```python
from build123d import *

# Parameters (mm, degrees)
SKETCH1_W           = 140
SKETCH1_H           = 70
BOSS_EXTRUDE1_DEPTH = 140
SKETCH2_W           = 134
SKETCH2_H           = 64
CUT_EXTRUDE1_DEPTH  = 133
SKETCH5_W           = 75.000260503
SKETCH5_H           = 36.846473491
BOSS_EXTRUDE3_DEPTH = 20
SKETCH6_W           = 5.75
SKETCH6_H           = 13
CUT_EXTRUDE2_DEPTH  = 3
SKETCH9_W           = 17
SKETCH9_H           = 30.85
CUT_EXTRUDE3_DEPTH  = 67
SKETCH11_W          = 140
SKETCH11_H          = 140
BOSS_EXTRUDE5_DEPTH = 5
SKETCH15_W          = 134
SKETCH15_H          = 4.072298399
CUT_EXTRUDE4_DEPTH  = 137


with BuildPart() as part:
    # Sketch1 → Boss-Extrude1 (new body)
    with BuildSketch(Plane(origin=(0, 0, 0), x_dir=(1, 0, 0), z_dir=(0, 1, 0))):
        with Locations((-46.886792453, 23.003144654)):
            Rectangle(SKETCH1_W, SKETCH1_H)
    extrude(amount=BOSS_EXTRUDE1_DEPTH)

    # Sketch2 → Cut-Extrude1 (cut)
    with BuildSketch(Plane(origin=(0, 140, 0), x_dir=(1, 0, 0), z_dir=(0, 1, 0))):
        with Locations((-46.932929257, 23.070074841)):
            Rectangle(SKETCH2_W, SKETCH2_H)
    extrude(amount=-CUT_EXTRUDE1_DEPTH, mode=Mode.SUBTRACT)

    # Sketch5 → Boss-Extrude3 (add)
    with BuildSketch(Plane.ZY.offset(116.886792453)):
        with Locations((-20.503014402, 18.423236746)):
            Rectangle(SKETCH5_W, SKETCH5_H)
    extrude(amount=BOSS_EXTRUDE3_DEPTH)

    # Sketch6 → Cut-Extrude2 (cut)
    with BuildSketch(Plane(origin=(0, 0, -58.003144654), x_dir=(-1, 0, 0), z_dir=(0, 0, -1))):
        with Locations((119.761792453, 20.746473491)):
            Rectangle(SKETCH6_W, SKETCH6_H)
    extrude(amount=-CUT_EXTRUDE2_DEPTH, mode=Mode.SUBTRACT)

    # Sketch9 → Cut-Extrude3 (cut)
    with BuildSketch(Plane.XY.offset(11.996855346)):
        with Locations((-125.382389836, 18.421473491)):
            Rectangle(SKETCH9_W, SKETCH9_H)
    extrude(amount=-CUT_EXTRUDE3_DEPTH, mode=Mode.SUBTRACT)

    # Sketch11 → Boss-Extrude5 (add)
    with BuildSketch(Plane.XY.offset(11.996855346)):
        with Locations((-46.886792453, 70)):
            Rectangle(SKETCH11_W, SKETCH11_H)
    extrude(amount=BOSS_EXTRUDE5_DEPTH)

    # Sketch15 → Cut-Extrude4 (cut)
    with BuildSketch(Plane(origin=(0, 140, 0), x_dir=(1, 0, 0), z_dir=(0, 1, 0))):
        with Locations((-46.932929257, -13.963840405)):
            Rectangle(SKETCH15_W, SKETCH15_H)
    extrude(amount=-CUT_EXTRUDE4_DEPTH, mode=Mode.SUBTRACT)


solid = part.part
```
Check sheet for the modelled part. Datum: model origin and axes. Units: mm. A direction names the side the tool comes from. Round coordinates to 2 decimals unless told otherwise and drop trailing zeros. Order: outer loops, then holes, each group sorted by start corner. A loop starts at its lowest first (then second) coordinate and runs counter-clockwise, first axis right, second up. Notation, with made-up numbers: (10, 32.25) - (54, 32.25) arc R11 cw to (54, 47.25) - close; hole circle Ø9 at (49.25, 82.5). An arc over 180 degrees is marked (long way). Write item = value, one per line.
Q1. Section check C-C (x = -93). Record the boundary of the cut face in (y, z), and give its area (3 significant figures).
Computed:
outline = (0, -58) - (140, -58) - (140, -55.07) - (7, -55.07) - (7, 8.93) - (140, 8.93) - (140, 11.93) - (3, 11.93) - (3, 16) - (140, 16) - (140, 17) - (0, 17) - close
area = 1,430 mm^2
Q2. Section check B-B (z = -27.5). Record the boundary of the cut face in (x, y), and give its area (3 significant figures).
Computed:
outline = (-136.89, 0) - (23.11, 0) - (23.11, 140) - (20.07, 140) - (20.07, 7) - (-113.93, 7) - (-113.93, 140) - (-116.89, 140) - (-116.89, 36.85) - (-136.89, 36.85) - close; hole (-133.88, 3) - (-116.88, 3) - (-116.88, 33.85) - (-133.88, 33.85) - close
area = 1,990 mm^2
Q3. Tool access check on faces 5 (the face through (-127, 19, -55.003)), 6 (the face through (-58, 0, -21)), 7 (the face through (-127, 36.846, -21)), 8 (the face through (20.067, 74, -23)), 9 (the face through (23.113, 69, -21)). Record the directions out of +Z, -Z, +X, -X, +Y, -Y that give a thin tool (end or side, any length) a straight path to the whole face; none if there is none.
Computed:
face_5 = none
face_6 = +Z, -Z, +X, -X, -Y
face_7 = +Z, -Z, -X, +Y
face_8 = +Y
face_9 = +Z, -Z, +X, +Y, -Y
Q4. Section check A-A (y = 47.5). Record the boundary of the cut face in (x, z), and give its area (3 significant figures).
Computed:
outline = (-116.89, -58) - (23.11, -58) - (23.11, 17) - (-116.89, 17) - close; hole (-113.93, -55.07) - (20.07, -55.07) - (20.07, 8.93) - (-113.93, 8.93) - close; hole (-113.93, 11.93) - (20.07, 11.93) - (20.07, 16) - (-113.93, 16) - close
area = 1,380 mm^2
Q5. Thickness scan on line 1 along Z through (x, y) = (-29, 88); line 2 along X through (y, z) = (12, -54.5); line 3 along X through (y, z) = (14, 11). Record the ranges inside material, lowest first.
Computed:
line_1 = -58 to -55.07, 8.93 to 11.93, 16 to 17
line_2 = -136.89 to -133.88, -116.88 to -113.93, 20.07 to 23.11
line_3 = -136.89 to -133.88, -116.88 to 23.11
Q6. Draft check along Y on faces 1 (the face through (-116.882, 18, -21)), 2 (the face through (-48, 7, -24)), 3 (the face through (-127, 18, 16.997)), 4 (the face through (-126, 33.846, -21)). Enter one of: pulls with the +Y half, pulls with the -Y half, needs draft (parallel to the pull), parting line crosses it, or undercut.
Computed:
face_1 = undercut
face_2 = pulls with the +Y half
face_3 = needs draft
face_4 = undercut
Q7. Go/stop test with flat-tipped pins: pin 1 (3.5 mm diameter, centred on x = -120, z = -57, fed in from +Y); pin 2 (19 mm diameter, centred on x = -32, z = -17.5, fed in from +Y); pin 3 (5 mm diameter, centred on y = 44.5, z = -1, fed in from -X). Record where each tip stops, or that it passes through.
Computed:
pin_1 = 36.85
pin_2 = 7
pin_3 = -116.89
